Geometry check sheet. Reference: the model listing, model coordinates, mm. Face numbers are marked on the shaded views. Give positions to 0.01 mm unless a question says otherwise; leave off trailing zeros. Write each loop counter-clockwise with the first axis right and the second up, starting at its lowest first coordinate (ties: lowest second). Pieces come first, ordered by that corner, then holes. Notation, with made-up numbers: M 77,87 L 108,87 A9 cw 108,91 Z; hole C 73,-7 d1. An arc over 180 degrees is marked long. One line per item, written item: value. Start each with the question number.
1. Cross-section at C-C on y = -3. Record the cut outline in (x, z), then the cut area to 3 significant figures.
2. Cross-section at D-D on y = -0.55. Record the cut outline in (x, z) (1 decimal).
3. Release check for a two-part mould opening along X. For the marked faces 1, 2 and 3 record: pulls with the +X half, pulls with the -X half, needs draft (parallel to the pull), parting line crosses it, or undercut.
4. Gauge pin test, flat ends, axial feed: pin 1 (1.5 mm diameter, centred on x = -1.5, z = -8, fed in from -Y); pin 2 (12 mm diameter, centred on x = 6.5, z = 4, fed in from +Y). Record the tip position at first contact, or that the pin passes through.
5. Scan lines: line 1 (Z direction, x = 0, y = -3.2); line 2 (Z direction, x = 8, y = -2.45); line 3 (Y direction, x = -7.25, z = 1). Record each from-to range of solid material in increasing order.
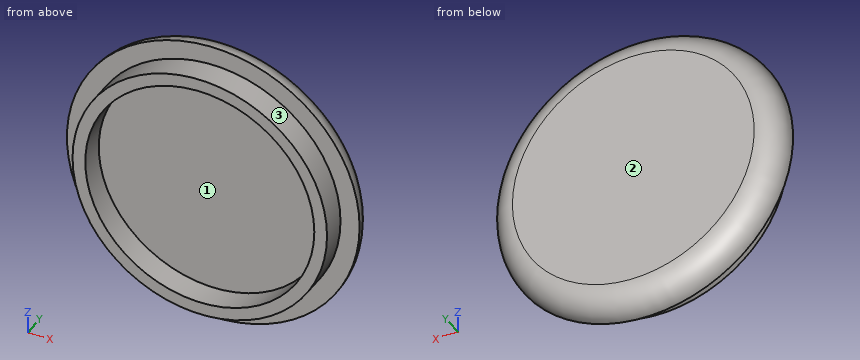
from build123d import *

# Parameters (mm, degrees)
F0_R     = 11.5
F1_DEPTH = 2
F2_R     = 10
F2_R_2   = 9
F3_DEPTH = 2
F4_R     = 1.99999


# Not quite as in the source:
# - a fillet or chamfer is up to 0.001 mm smaller than in the source, because OpenCascade refuses the exact size


with BuildPart() as f1:
    # F0 (on Front) → F1 (new body)
    with BuildSketch(Plane.XZ):
        Circle(F0_R)
    extrude(amount=F1_DEPTH)

    # F2 (on face) → F3 (join)
    with BuildSketch(Plane.XZ.offset(2)):
        Circle(F2_R)
        Circle(F2_R_2, mode=Mode.SUBTRACT)
    extrude(amount=F3_DEPTH)

    # F4 (radius 2 in the source; OpenCascade refuses exactly that, so slightly less here)
    f4_edges = [f1.edges().sort_by_distance(p)[0] for p in [
        (-11.5, 0, 0),
    ]]
    fillet(f4_edges, radius=F4_R)


solid = f1.part
Report:
1. outline: C 0,0 d20; hole C 0,0 d18
1. area: 59.7 mm^2
2. outline: C 0,0 d21.8
3. face 1: undercut
3. face 2: needs draft
3. face 3: parting line crosses it
4. pin 1: stops at y = -2
4. pin 2: stops at y = 0
5. line 1: z = -10 to -9, 9 to 10
5. line 2: z = -6 to -4.12, 4.12 to 6
5. line 3: y = -2 to 0
